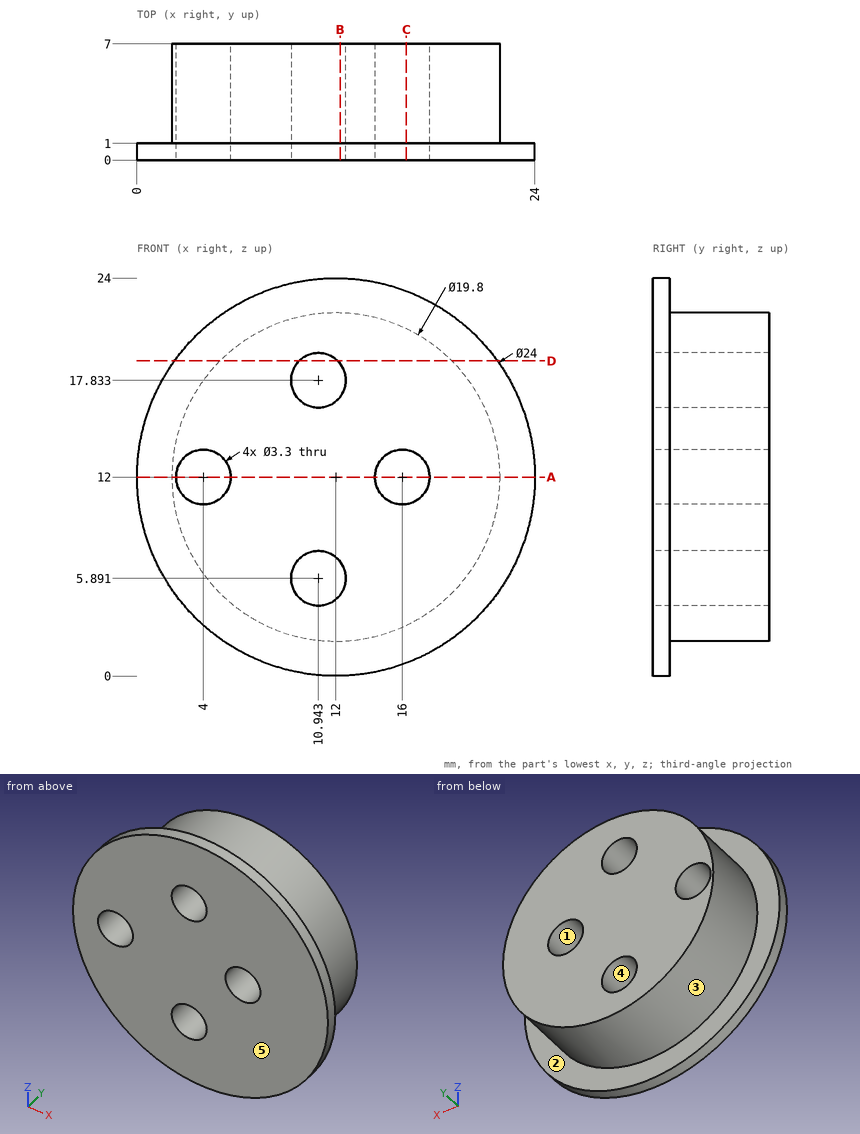
Study the drawing (mm; zero at the part's minimum x, y, z) and answer. A direction names the side the tool comes from. Coordinates: 2 decimals unless noted, no trailing zeros. Write each loop counter-clockwise with the first axis right and the second up, starting at its lowest first coordinate (ties: lowest second). Pieces come first, ordered by that corner, then holes. Notation, with made-up numbers: M -18,49 L 21,49 A20 ccw 21,53 Z; hole C 52.25,0.25 d10. An arc over 180 degrees is marked long. Use a Markdown table: item, result. Add a question column.
1. Which of the six approach directions +Z, -Z, +X, -X, +Y, -Y give full straight-line access (tool end or side, diameter ignored) to the marked faces 1 and 2?
2. Section A-A (z = 12) is taken. Give the vertices of the cut face in (x, y).
3. Section D-D (z = 19) is taken. Give the vertices of the cut face in (x, y).
4. Section B-B (x = 12.25) is taken. Give the vertices of the cut face in (y, z) (1 decimal).
5. For a pull along X with two mould halves and no side action, classify the marked faces 3, 4 and 5 as +X half, -X half, draft (parallel to the pull), parting line (faces both ways), or undercut.
6. Given P1, Ø2, axis at y = 5.5, z = 7, coming from the -X side (1 decimal); P2, Ø2, axis at y = 3.5, z = 5, coming from the +X side (1 decimal), each flat-ended and moving along its own axis, determine where each tip first touches the part or whether it passes through.
7. Straight lines are drawn through the part: line 1 along X through (y, z) = (4.5, 12); line 2 along Z through (x, y) = (10.75, 2.75) (1 decimal); line 3 along X through (y, z) = (5.5, 12.75). For each, find the intervals that lie inside material, in ascending order. Write a range as [from, to].
8. Section C-C (x = 16.25) is taken. Give the vertices of the cut face in (y, z), plus the area to 3 significant figures.
Data:
| question | item | result |
|---|---|---|
| 1 | face 1 | +Y, -Y |
| 1 | face 2 | +Y |
| 2 | outline | M 0,0 L 2.35,0 L 2.35,7 L 2.1,7 L 2.1,1 L 0,1 Z; M 5.65,0 L 14.35,0 L 14.35,7 L 5.65,7 Z; M 17.65,0 L 24,0 L 24,1 L 21.9,1 L 21.9,7 L 17.65,7 Z |
| 3 | outline | M 2.25,0 L 9.78,0 L 9.78,7 L 5,7 L 5,1 L 2.25,1 Z; M 12.11,0 L 21.75,0 L 21.75,1 L 19,1 L 19,7 L 12.11,7 Z |
| 4 | outline | M 0,0 L 1,0 L 1,2.1 L 7,2.1 L 7,4.9 L 0,4.9 Z; M 0,6.9 L 7,6.9 L 7,16.8 L 0,16.8 Z; M 0,18.8 L 7,18.8 L 7,21.9 L 1,21.9 L 1,24 L 0,24 Z |
| 5 | face 3 | parting line |
| 5 | face 4 | undercut |
| 5 | face 5 | draft |
| 6 | P1 | stops at x = 2.9 |
| 6 | P2 | stops at x = 19.9 |
| 7 | line 1 | x = [2.1, 2.35], [5.65, 14.35], [17.65, 21.9] |
| 7 | line 2 | z = [2.2, 4.3], [7.5, 16.2], [19.5, 21.8] |
| 7 | line 3 | x = [2.13, 2.53], [5.47, 14.53], [17.47, 21.87] |
| 8 | outline | M 0,0.78 L 1,0.78 L 1,3.06 L 7,3.06 L 7,10.37 L 0,10.37 Z; M 0,13.63 L 7,13.63 L 7,20.94 L 1,20.94 L 1,23.22 L 0,23.22 Z |
| 8 | area | 107 mm2 |
